```python
from build123d import *

# Parameters (mm, degrees)
BOSS_EXTRUDE2_DEPTH = 30
FILLET2_R           = 2
BOSS_EXTRUDE3_DEPTH = 30
SKETCH5_R           = 1.5
BOSS_EXTRUDE4_DEPTH = 30


with BuildPart() as part:
    # Sketch1 → Boss-Extrude2 (new body)
    with BuildSketch(Plane.XY):
        Polygon((4, 4), (-35.712592027, 4), (4, -105.109449862), align=None)
        Polygon((0, 0), (-30, 0), (-27.088238126, -8), (0, -8), align=None, mode=Mode.SUBTRACT)
        Polygon((0, -82.424322584), (0, -69.4), (-4.740465742, -69.4), align=None, mode=Mode.SUBTRACT)
        Polygon((-26.578679798, -9.4), (0, -9.4), (0, -18), (-23.448535783, -18), align=None, mode=Mode.SUBTRACT)
        Polygon((-22.938977455, -19.4), (0, -19.4), (0, -28), (-19.808833441, -28), align=None, mode=Mode.SUBTRACT)
        Polygon((-19.299275113, -29.4), (0, -29.4), (0, -38), (-16.169131098, -38), align=None, mode=Mode.SUBTRACT)
        Polygon((-15.65957277, -39.4), (0, -39.4), (0, -48), (-12.529428755, -48), align=None, mode=Mode.SUBTRACT)
        Polygon((-12.019870427, -49.4), (0, -49.4), (0, -58), (-8.889726413, -58), align=None, mode=Mode.SUBTRACT)
        Polygon((-8.380168085, -59.4), (0, -59.4), (0, -68), (-5.25002407, -68), align=None, mode=Mode.SUBTRACT)
    extrude(amount=BOSS_EXTRUDE2_DEPTH)

    # Fillet2
    fillet2_edges = [part.edges().sort_by_distance(p)[0] for p in [
        (-35.712592027, 4, 15),
        (4, 4, 15),
        (4, -105.109449862, 15),
    ]]
    fillet(fillet2_edges, radius=FILLET2_R)

    # Sketch4 → Boss-Extrude3 (add)
    with BuildSketch(Plane.XY.offset(30)):
        with BuildLine():
            Line((-14.90441672, -26.3), (-4.90441672, -26.3))
            ThreePointArc((-4.90441672, -26.3), (-2.50441672, -28.7), (-4.90441672, -31.1))
            Line((-4.90441672, -31.1), (-14.90441672, -31.1))
            ThreePointArc((-14.90441672, -31.1), (-17.30441672, -28.7), (-14.90441672, -26.3))
        make_face()
        with BuildLine():
            Line((-4.084565549, -41.1), (-12.084565549, -41.1))
            ThreePointArc((-12.084565549, -41.1), (-14.484565549, -38.7), (-12.084565549, -36.3))
            Line((-12.084565549, -36.3), (-4.084565549, -36.3))
            ThreePointArc((-4.084565549, -36.3), (-1.684565549, -38.7), (-4.084565549, -41.1))
        make_face()
        with BuildLine():
            Line((-8.764714378, -46.3), (-3.764714378, -46.3))
            ThreePointArc((-3.764714378, -46.3), (-1.364714378, -48.7), (-3.764714378, -51.1))
            Line((-3.764714378, -51.1), (-8.764714378, -51.1))
            ThreePointArc((-8.764714378, -51.1), (-11.164714378, -48.7), (-8.764714378, -46.3))
        make_face()
        with BuildLine():
            Line((-4.944863206, -56.3), (-3.944863206, -56.3))
            ThreePointArc((-3.944863206, -56.3), (-1.544863206, -58.7), (-3.944863206, -61.1))
            Line((-3.944863206, -61.1), (-4.944863206, -61.1))
            ThreePointArc((-4.944863206, -61.1), (-7.344863206, -58.7), (-4.944863206, -56.3))
        make_face()
        with BuildLine():
            Line((-5.724267892, -21.1), (-17.724267892, -21.1))
            ThreePointArc((-17.724267892, -21.1), (-20.124267892, -18.7), (-17.724267892, -16.3))
            Line((-17.724267892, -16.3), (-5.724267892, -16.3))
            ThreePointArc((-5.724267892, -16.3), (-3.324267892, -18.7), (-5.724267892, -21.1))
        make_face()
    extrude(amount=-BOSS_EXTRUDE3_DEPTH)

    # Sketch5 → Boss-Extrude4 (add)
    with BuildSketch(Plane.XY.offset(30)):
        with Locations((-2.625012035, -68.7)):
            Circle(SKETCH5_R)
    extrude(amount=-BOSS_EXTRUDE4_DEPTH)


solid = part.part
```
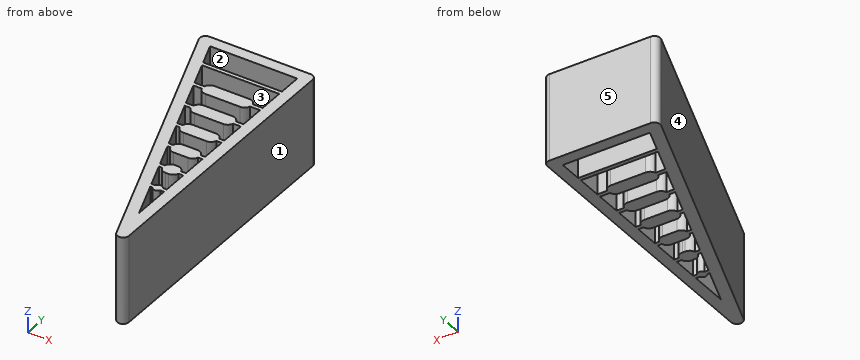
Check sheet for the modelled part. Datum: model origin and axes. Units: mm. Face numbers are marked on the shaded views. A direction names the side the tool comes from. Coordinates: 2 decimals unless noted, no trailing zeros. Order: outer loops, then holes, each group sorted by start corner. A loop starts at its lowest first (then second) coordinate and runs counter-clockwise, first axis right, second up. Notation, with made-up numbers: (-16.5, 0) -> (-12.5, 0) arc R19 cw to (-12.5, 14) -> close; hole circle Ø10 at (-28.75, 27.5). An arc over 180 degrees is marked (long way). Write item = value, one per line. Start each with the question number.
1) Access from +Z, -Z, +X, -X, +Y, -Y to the whole of each face (thin tool, end or side, straight path). Record for the marked faces 1 and 2.
2) Material ranges on L1, parallel to X at y = -16.5, z = 11.75; L2, parallel to X at y = -26.5, z = 9.25; L3, parallel to X at y = -7, z = 26.75, recorded low to high.
3) Mould release check, pull along Y, two halves, no side actions. Record for the marked faces 3, 4 and 5: +Y half, -Y half, draft (parallel to the pull), parting line (faces both ways), or undercut.
4) Cross-section at A-A (x = -21). Enter the section's corners in (y, z).
5) Cross-section at C-C (x = -10). Enter the section's corners in (y, z).
6) Cross-section at D-D (z = 26.75). State how many separate pieces and enclosed holes the cut face has, then the cut area to 3 significant figures.
7) Cross-section at B-B (y = -77). Enter the section's corners in (x, z).
8) Go/stop test with flat-tipped pins: P1, Ø2, axis at y = -77, z = 12, coming from the -X side (3 decimals); P2, Ø10, axis at y = -30.5, z = 16, coming from the -X side; P3, Ø7, axis at y = -42.5, z = 21.5, coming from the -X side. Record where each tip stops, or that it passes through.
Ans:
q1.face_1 = +Z, -Z, +X, +Y, -Y
q1.face_2 = +Z, -Z
q2.L1 = -28.25 to -23.99, -18.68 to -4.77, 0 to 4
q2.L2 = -24.61 to -20.35, -15.86 to -3.95, 0 to 4
q2.L3 = -31.71 to -27.45, 0 to 4
q3.face_3 = undercut
q3.face_4 = -Y half
q3.face_5 = +Y half
q4.outline = (-36.42, 0) -> (-24.73, 0) -> (-24.73, 30) -> (-36.42, 30) -> close; (-19.4, 0) -> (-18, 0) -> (-18, 30) -> (-19.4, 30) -> close; (-9.4, 0) -> (-8, 0) -> (-8, 30) -> (-9.4, 30) -> close; (0, 0) -> (4, 0) -> (4, 30) -> (0, 30) -> close
q5.outline = (-66.64, 0) -> (-54.95, 0) -> (-54.95, 30) -> (-66.64, 30) -> close; (-50.76, 0) -> (-46.64, 0) -> (-46.64, 30) -> (-50.76, 30) -> close; (-41.1, 0) -> (-36.3, 0) -> (-36.3, 30) -> (-41.1, 30) -> close; (-31.1, 0) -> (-26.3, 0) -> (-26.3, 30) -> (-31.1, 30) -> close; (-21.1, 0) -> (-16.3, 0) -> (-16.3, 30) -> (-21.1, 30) -> close; (-9.4, 0) -> (-8, 0) -> (-8, 30) -> (-9.4, 30) -> close; (0, 0) -> (4, 0) -> (4, 30) -> (0, 30) -> close
q6.separate_pieces = 1
q6.enclosed_holes = 8
q6.area = 1,250 mm²
q7.outline = (-6.23, 0) -> (-1.97, 0) -> (-1.97, 30) -> (-6.23, 30) -> close; (0, 0) -> (4, 0) -> (4, 30) -> (0, 30) -> close
q8.P1 = -6.595
q8.P2 = -24.98
q8.P3 = -20.06
